CAD build for the part. Positions are in the model's coordinates, mm. A direction names the side the tool comes from. Round coordinates to 2 decimals unless told otherwise and drop trailing zeros. Loops run counter-clockwise (first coordinate to the right, second up) from the corner with the lowest first, then second, coordinate; pieces in that order, holes last.
```python
from build123d import *

# Parameters (mm, degrees)
BOSS_EXTRUDE1_DEPTH      = 52
BOSS_EXTRUDE1_DEPTH_BACK = 52
SKETCH1_W                = 120
SKETCH1_H                = 4
BOSS_EXTRUDE2_START      = -20
SKETCH1_3_R              = 4
BOSS_EXTRUDE2_DEPTH      = 6
LPATTERN1_COUNT          = 2
LPATTERN1_PITCH          = 21
BOSS_EXTRUDE3_START      = -15.5
SKETCH1_4_R              = 4.1
BOSS_EXTRUDE3_DEPTH      = 6
SKETCH2_R                = 4
SKETCH2_W                = 15.5
SKETCH2_H                = 74.282546786
SKETCH2_H_2              = 13.357231507
CUT_EXTRUDE1_DEPTH       = 96.858544882
MIRROR2_START            = -20
MIRROR2_COPY_1_SKETCH_R  = 4
MIRROR2_COPY_1_DEPTH     = 6
SKETCH4_R                = 3
CUT_EXTRUDE2_DEPTH       = 10
SKETCH5_W                = 11
SKETCH5_H                = 22
SKETCH5_W_2              = 15
SKETCH5_H_2              = 15.5
SKETCH5_W_3              = 28
SKETCH5_H_3              = 24.360221707
CUT_EXTRUDE3_DEPTH       = 10
FILLET1_R                = 6
FILLET2_R                = 3
FILLET3_R                = 5


with BuildPart() as part:
    # Sketch1 → Boss-Extrude1 (new, two sides: drawn at the far end of the back side and taken through both)
    with BuildSketch(Plane(origin=(0, 0, 0), x_dir=(0, 0, -1), z_dir=(1, 0, 0)).offset(-BOSS_EXTRUDE1_DEPTH_BACK)):
        with Locations((-16.322496103, -16.524005043)):
            Rectangle(SKETCH1_W, SKETCH1_H)
    extrude(amount=BOSS_EXTRUDE1_DEPTH + BOSS_EXTRUDE1_DEPTH_BACK)

    # Sketch1_3 → Boss-Extrude2 (add)
    with BuildSketch(Plane(origin=(0, 0, 0), x_dir=(0, 0, -1), z_dir=(1, 0, 0)).offset(BOSS_EXTRUDE2_START)):
        with BuildLine():
            Line((-54.601909319, 4.550530592), (-57.965264596, -14.524005043))
            Line((-57.965264596, -14.524005043), (-35.605042889, -14.524005043))
            Line((-35.605042889, -14.524005043), (-38.723447295, 3.161345171))
            ThreePointArc((-38.723447295, 3.161345171), (-46.026201353, 11.130902756), (-54.601909319, 4.550530592))
        make_face()
        with Locations((-46.723447295, 3.161345171)):
            Circle(SKETCH1_3_R, mode=Mode.SUBTRACT)
    boss_extrude2 = extrude(amount=-BOSS_EXTRUDE2_DEPTH)

    # LPattern1: Boss-Extrude2 ×2
    with Locations(*[(-i * LPATTERN1_PITCH, 0, 0) for i in range(1, LPATTERN1_COUNT)]):
        add(boss_extrude2)

    # Sketch1_4 → Boss-Extrude3 (add)
    with BuildSketch(Plane(origin=(0, 0, 0), x_dir=(0, 0, -1), z_dir=(1, 0, 0)).offset(BOSS_EXTRUDE3_START)):
        Polygon((14.677503897, -14.524005043), (20.501027646, 1.475994957), (32.853980149, 1.475994957), (38.677503897, -14.524005043), align=None)
        with Locations((26.677503897, -6.524005043)):
            Circle(SKETCH1_4_R, mode=Mode.SUBTRACT)
    boss_extrude3 = extrude(amount=-BOSS_EXTRUDE3_DEPTH)

    # Sketch2 → Cut-Extrude1 (cut, through all)
    with BuildSketch(Plane(origin=(0, -14.524005043, 0), x_dir=(1, 0, 0), z_dir=(0, 1, 0))):
        with Locations(Location((-33.5, -67.322496103, 0), (0, 0, 270))):
            Circle(SKETCH2_R)
        with Locations(Location((-33.5, 34.677503897, 0), (0, 0, 270))):
            Circle(SKETCH2_R)
        Polygon((-52, -76.322496103), (-40, -76.322496103), (-52, -64.322496103), align=None)
        Polygon((-42.5, 43.677503897), (-42.5, -11.105042889), (-52, -20.605042889), (-52, 43.677503897), align=None)
        with Locations((-7.75, 6.536230504)):
            Rectangle(SKETCH2_W, SKETCH2_H)
        with Locations((-7.75, -69.64388035)):
            Rectangle(SKETCH2_W, SKETCH2_H_2)
    cut_extrude1 = extrude(amount=-CUT_EXTRUDE1_DEPTH, mode=Mode.SUBTRACT)

    # Mirror2: Boss-Extrude2, Boss-Extrude3, Cut-Extrude1 across plane
    add(boss_extrude2.mirror(Plane(origin=(0, 0, 0), x_dir=(0, 0, 1), z_dir=(1, 0, 0))))
    add(boss_extrude3.mirror(Plane(origin=(0, 0, 0), x_dir=(0, 0, 1), z_dir=(1, 0, 0))))
    add(cut_extrude1.mirror(Plane(origin=(0, 0, 0), x_dir=(0, 0, 1), z_dir=(1, 0, 0))), mode=Mode.SUBTRACT)

    # Mirror2 copy 1 sketch → Mirror2 copy 1 (add)
    with BuildSketch(Plane(origin=(21, 0, 0), x_dir=(0, 0, -1), z_dir=(-1, 0, 0)).offset(MIRROR2_START)):
        with BuildLine():
            Line((-54.601909319, -4.550530592), (-57.965264596, 14.524005043))
            Line((-57.965264596, 14.524005043), (-35.605042889, 14.524005043))
            Line((-35.605042889, 14.524005043), (-38.723447295, -3.161345171))
            ThreePointArc((-38.723447295, -3.161345171), (-46.026201353, -11.130902756), (-54.601909319, -4.550530592))
        make_face()
        with Locations((-46.723447295, -3.161345171)):
            Circle(MIRROR2_COPY_1_SKETCH_R, mode=Mode.SUBTRACT)
    extrude(amount=-MIRROR2_COPY_1_DEPTH)

    # Sketch4 → Cut-Extrude2 (cut)
    with BuildSketch(Plane(origin=(0, -14.524005043, 0), x_dir=(1, 0, 0), z_dir=(0, 1, 0))):
        with Locations(Location((22, -8.064569544, 0), (0, 0, 270))):
            Circle(SKETCH4_R)
        with Locations(Location((-22, -8.064569544, 0), (0, 0, 270))):
            Circle(SKETCH4_R)
    extrude(amount=-CUT_EXTRUDE2_DEPTH, mode=Mode.SUBTRACT)

    # Sketch5 → Cut-Extrude3 (cut)
    with BuildSketch(Plane(origin=(0, -14.524005043, 0), x_dir=(1, 0, 0), z_dir=(0, 1, 0))):
        with Locations((-32, 11.894957111)):
            Rectangle(SKETCH5_W, SKETCH5_H)
        with Locations((-33.5, -23.855042889)):
            Rectangle(SKETCH5_W_2, SKETCH5_H_2)
        with Locations((0, -46.785153743)):
            Rectangle(SKETCH5_W_3, SKETCH5_H_3)
        with Locations((33.5, -23.855042889)):
            Rectangle(SKETCH5_W_2, SKETCH5_H_2)
        with Locations((32, 11.894957111)):
            Rectangle(SKETCH5_W, SKETCH5_H)
    extrude(amount=-CUT_EXTRUDE3_DEPTH, mode=Mode.SUBTRACT)

    # Fillet1
    fillet1_edges = [part.edges().sort_by_distance(p)[0] for p in [
        (-52, -16.524005043, 64.322496103),
        (-40, -16.524005043, 76.322496103),
        (-15.5, -16.524005043, 76.322496103),
        (-15.5, -16.524005043, 62.965264596),
        (15.5, -16.524005043, -43.677503897),
        (15.5, -16.524005043, 30.605042889),
        (42.5, -16.524005043, -43.677503897),
        (52, -16.524005043, 20.605042889),
        (42.5, -16.524005043, 11.105042889),
        (52, -16.524005043, 64.322496103),
        (40, -16.524005043, 76.322496103),
        (15.5, -16.524005043, 62.965264596),
        (15.5, -16.524005043, 76.322496103),
        (-15.5, -16.524005043, 30.605042889),
        (-15.5, -16.524005043, -43.677503897),
        (-42.5, -16.524005043, -43.677503897),
        (-42.5, -16.524005043, 11.105042889),
        (-52, -16.524005043, 20.605042889),
    ]]
    fillet(fillet1_edges, radius=FILLET1_R)

    # Fillet2
    fillet2_edges = [part.edges().sort_by_distance(p)[0] for p in [
        (26.5, -16.524005043, -0.894957111),
        (26.5, -16.524005043, -22.894957111),
        (37.5, -16.524005043, -22.894957111),
        (37.5, -16.524005043, -0.894957111),
        (41, -16.524005043, 31.605042889),
        (26, -16.524005043, 31.605042889),
        (26, -16.524005043, 16.105042889),
        (41, -16.524005043, 16.105042889),
        (14, -16.524005043, 34.605042889),
        (14, -16.524005043, 58.965264596),
        (-14, -16.524005043, 58.965264596),
        (-14, -16.524005043, 34.605042889),
        (-26, -16.524005043, 31.605042889),
        (-41, -16.524005043, 31.605042889),
        (-41, -16.524005043, 16.105042889),
        (-26, -16.524005043, 16.105042889),
        (-37.5, -16.524005043, -0.894957111),
        (-37.5, -16.524005043, -22.894957111),
        (-26.5, -16.524005043, -22.894957111),
        (-26.5, -16.524005043, -0.894957111),
    ]]
    fillet(fillet2_edges, radius=FILLET2_R)

    # Fillet3
    fillet3_edges = [part.edges().sort_by_distance(p)[0] for p in [
        (-44, -14.524005043, 57.965264596),
        (-23, -14.524005043, 57.965264596),
        (23, -14.524005043, 57.965264596),
        (44, -14.524005043, 57.965264596),
        (-44, -14.524005043, 35.605042889),
        (-23, -14.524005043, 35.605042889),
        (23, -14.524005043, 35.605042889),
        (44, -14.524005043, 35.605042889),
        (-18.5, 1.475994957, -20.501027646),
        (-18.5, -14.524005043, -14.677503897),
        (-18.5, 1.475994957, -32.853980149),
        (-18.541960108, -14.524005043, -38.677503897),
        (18.541960108, -14.524005043, -38.677503897),
        (18.5, 1.475994957, -32.853980149),
        (18.5, 1.475994957, -20.501027646),
        (18.5, -14.524005043, -14.677503897),
    ]]
    fillet(fillet3_edges, radius=FILLET3_R)


solid = part.part
```
Item 1: Cut at B-B, the plane z = 53. Give the cut face in (x, y).
Answers follow:
outline: (-52, -18.52) - (-14, -18.52) - (-14, -14.52) - (-20, -14.52) - (-20, 8.12) - (-26, 8.12) - (-26, -14.52) - (-41, -14.52) - (-41, 8.12) - (-47, 8.12) - (-47, -14.52) - (-52, -14.52) - close; (14, -18.52) - (52, -18.52) - (52, -14.52) - (47, -14.52) - (47, 8.12) - (41, 8.12) - (41, -14.52) - (26, -14.52) - (26, 8.12) - (20, 8.12) - (20, -14.52) - (14, -14.52) - close
Item 2: Cut at C-C, the plane x = 31. Give the cut face in (y, z) (1 decimal).
Answers follow:
outline: (-18.5, -43.7) - (-14.5, -43.7) - (-14.5, -37.8) - (-18.5, -37.8) - close; (-18.5, -31.6) - (-14.5, -31.6) - (-14.5, -22.9) - (-18.5, -22.9) - close; (-18.5, -0.9) - (-14.5, -0.9) - (-14.5, 16.1) - (-18.5, 16.1) - close; (-18.5, 31.6) - (-14.5, 31.6) - (-14.5, 64.2) - (-18.5, 64.2) - close; (-18.5, 70.4) - (-14.5, 70.4) - (-14.5, 76.3) - (-18.5, 76.3) - close
Item 3: Cut at D-D, the plane z = 21. Give the cut face in (x, y), plus the area to 3 significant figures.
Answers follow:
outline: (-51.62, -18.52) - (-41, -18.52) - (-41, -14.52) - (-51.62, -14.52) - close; (-26, -18.52) - (-15.5, -18.52) - (-15.5, -14.52) - (-26, -14.52) - close; (15.5, -18.52) - (26, -18.52) - (26, -14.52) - (15.5, -14.52) - close; (41, -18.52) - (51.62, -18.52) - (51.62, -14.52) - (41, -14.52) - close
area: 169 mm2
Item 4: Cut at A-A, the plane x = 4.5. Give the cut face in (y, z), plus the area to 3 significant figures.
Answers follow:
outline: (-18.52, 30.61) - (-14.52, 30.61) - (-14.52, 34.61) - (-18.52, 34.61) - close; (-18.52, 58.97) - (-14.52, 58.97) - (-14.52, 62.97) - (-18.52, 62.97) - close
area: 32.0 mm2
Item 5: 3-axis set-ups, long thin cutter, end or side, ignore diameter. For faces 5 (the cylindrical face through (-18.542, -13.644, -39.346)), 6 (the flat face through (41, -16, 24)): which of +Z, -Z, +X, -X, +Y, -Y reach the whole face in a straight line?
Answers follow:
face 5: -Z, +X, -X, +Y
face 6: +Y, -Y
Item 6: Two-plate mould, pull along Z, no slides. Class faces 1 (the cylindrical face through (-40.1, -16.55, 16.96)), 2 (the flat face through (-26, -4, 47)), 3 (the cylindrical face through (40.79, -16.55, -41.87)), 4 (the cylindrical face through (22.958, 4.363, 42.908)): released by +Z, released by -Z, zero draft, split by the parting line, or undercut.
Answers follow:
face 1: undercut
face 2: zero draft
face 3: released by -Z
face 4: undercut
Item 7: Flat gauge pins, fed straight in: P1, Ø3.5, axis at x = 22, z = 8.06, coming from the +Y side; P2, Ø12, axis at x = 22.5, y = 5.5, coming from the +Z side; P3, Ø4, axis at x = -32.5, z = 61.5, coming from the +Y side; P4, Ø1.5, axis at y = -16.5, z = 70, coming from the +X side. Where does each tip first touch, or does it go through?
Answers follow:
P1: passes through
P2: stops at z = 55.49
P3: stops at y = -14.52
P4: stops at x = 47.07
Item 8: Probe line 1 (X direction, y = -16.75, z = -13); line 2 (X direction, y = -1.25, z = 49.5); line 3 (Z direction, x = 37, y = -15.25). List the from-to ranges inside material, lowest first.
Answers follow:
line 1: x = -42.5 to -37.5, -26.5 to -15.5, 15.5 to 26.5, 37.5 to 42.5
line 2: x = -47 to -41, -26 to -20, 20 to 26, 41 to 47
line 3: z = -43.66 to -36.61, -32.74 to -21.55, -2.24 to 16.11, 31.61 to 65.39, 69.26 to 76.32
